from build123d import *

# Parameters (mm, degrees)
F1_DEPTH = 3


with BuildPart() as f1:
    # F0 (on Top) → F1 (new body)
    with BuildSketch(Plane.XY):
        with BuildLine():
            ThreePointArc((0, 8.660254), (-15, 0), (0, -8.660254))
            ThreePointArc((0, -8.660254), (15, 0), (0, 8.660254))
        make_face()
        with BuildLine():
            ThreePointArc((-0.95, 8.037257), (-3.930286, 4.5), (-5, 0))
            ThreePointArc((-5, 0), (-3.930286, -4.5), (-0.95, -8.037257))
            ThreePointArc((-0.95, -8.037257), (-14, 0), (-0.95, 8.037257))
        make_face(mode=Mode.SUBTRACT)
        with BuildLine():
            ThreePointArc((0, -7.483315), (-2.937254, -4.242641), (-4, 0))
            ThreePointArc((-4, 0), (-2.937254, 4.242641), (0, 7.483315))
            ThreePointArc((0, 7.483315), (2.937254, 4.242641), (4, 0))
            ThreePointArc((4, 0), (2.937254, -4.242641), (0, -7.483315))
        make_face(mode=Mode.SUBTRACT)
        with BuildLine():
            ThreePointArc((0.95, -8.037257), (3.930286, -4.5), (5, 0))
            ThreePointArc((5, 0), (3.930286, 4.5), (0.95, 8.037257))
            ThreePointArc((0.95, 8.037257), (14, 0), (0.95, -8.037257))
        make_face(mode=Mode.SUBTRACT)
    extrude(amount=F1_DEPTH)


solid = f1.part
Geometry: final body of the model. Coordinates: model frame, mm. Give positions to 0.01 mm unless a question says otherwise; leave off trailing zeros. Write each loop counter-clockwise with the first axis right and the second up, starting at its lowest first coordinate (ties: lowest second). Pieces come first, ordered by that corner, then holes.
(1) Ray query, line 1 (X direction, y = -1.5, z = 2.05); line 2 (X direction, y = 7.25, z = 1.45); line 3 (Y direction, x = -8, z = 1.9). Return the intervals inside material, ascending.
(2) First-contact query: P1, Ø1, axis at x = -10.5, z = 1, coming from the -Y side. Flat tip, straight axial feed; report the tip coordinate or a pass-through.
(3) Cut plane A-A, the plane x = -9. Return loops of the section in (y, z).
(4) Cut plane D-D, the plane x = 12.5. Return loops of the section in (y, z), then the cut area to 3 significant figures.
(5) Cut plane B-B, the plane z = 0.8. Return loops of the section in (x, y), then the cut area to 3 significant figures.
(6) Mould query, pull axis Y, two halves, no side actions, for faces 1 (the cylindrical face through (-14, 0, 1)), 2 (the flat face through (-4.5, 0.8, 0)), 3 (the cylindrical face through (15, 0, 1)). Classes: released by +Y, released by -Y, zero draft, split by the parting line, or undercut.
(7) Cut plane C-C, the plane x = 3.5. Return loops of the section in (y, z).
Values follow:
1. line 1: x = -14.89 to -13.87, -4.89 to -3.87, 3.87 to 4.89, 13.87 to 14.89
1. line 2: x = -11.89 to -10.33, -1.89 to -0.33, 0.33 to 1.89, 10.33 to 11.89
1. line 3: y = -9.54 to -8.49, 8.49 to 9.54
2. P1: stops at y = -8.66
3. outline: (-9.17, 0) - (-8.06, 0) - (-8.06, 3) - (-9.17, 3) - close; (8.06, 0) - (9.17, 0) - (9.17, 3) - (8.06, 3) - close
4. outline: (-6.61, 0) - (-4.97, 0) - (-4.97, 3) - (-6.61, 3) - close; (4.97, 0) - (6.61, 0) - (6.61, 3) - (4.97, 3) - close
4. area: 9.84 mm2
5. outline: (0, -8.66) arc R10 ccw (long way) to (0, 8.66) arc R10 ccw (long way) to start; hole (-5, 0) arc R10 cw to (-0.95, 8.04) arc R9 ccw (long way) to (-0.95, -8.04) arc R10 cw to start; hole (-4, 0) arc R9 ccw to (0, -7.48) arc R9 ccw to (4, 0) arc R9 ccw to (0, 7.48) arc R9 ccw to start; hole (0.95, -8.04) arc R9 ccw (long way) to (0.95, 8.04) arc R10 cw to (5, 0) arc R10 cw to start
5. area: 117 mm2
6. face 1: undercut
6. face 2: zero draft
6. face 3: split by the parting line
7. outline: (-9.89, 0) - (-8.87, 0) - (-8.87, 3) - (-9.89, 3) - close; (-5.27, 0) - (-2.96, 0) - (-2.96, 3) - (-5.27, 3) - close; (2.96, 0) - (5.27, 0) - (5.27, 3) - (2.96, 3) - close; (8.87, 0) - (9.89, 0) - (9.89, 3) - (8.87, 3) - close
